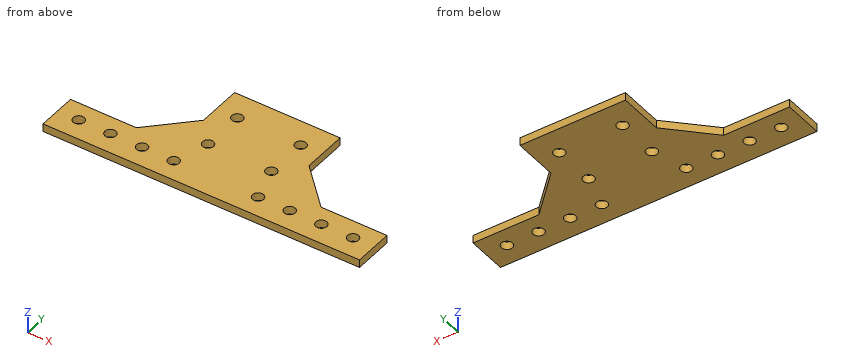
```python
from build123d import *

# Parameters (mm, degrees)
EXTRUDE_1_DEPTH     = 3
SKETCH_2_R          = 2.1
CUT_EXTRUDE_1_DEPTH = 129.910821889


with BuildPart() as part:
    # 草图1 → 凸台-拉伸1 (new body)
    with BuildSketch(Plane.XY):
        Polygon((0, 0), (0, 15), (25, 15), (40, 30), (40, 47), (80, 47), (80, 30), (95, 15), (120, 15), (120, 0), align=None)
    extrude(amount=EXTRUDE_1_DEPTH)

    # 草图2 → 切除-拉伸1 (cut, through all)
    with BuildSketch(Plane.XY.offset(3)):
        with Locations((48, 37)):
            Circle(SKETCH_2_R)
        with Locations((72, 37)):
            Circle(SKETCH_2_R)
        with Locations((48, 21)):
            Circle(SKETCH_2_R)
        with Locations((72, 21)):
            Circle(SKETCH_2_R)
        with Locations((112, 8)):
            Circle(SKETCH_2_R)
        with Locations((76, 8)):
            Circle(SKETCH_2_R)
        with Locations((88, 8)):
            Circle(SKETCH_2_R)
        with Locations((8, 8)):
            Circle(SKETCH_2_R)
        with Locations((20, 8)):
            Circle(SKETCH_2_R)
        with Locations((100, 8)):
            Circle(SKETCH_2_R)
        with Locations((32, 8)):
            Circle(SKETCH_2_R)
        with Locations((44, 8)):
            Circle(SKETCH_2_R)
        with Locations((432, 8)):
            Circle(SKETCH_2_R)
        with Locations((444, 8)):
            Circle(SKETCH_2_R)
        with Locations((524, 8)):
            Circle(SKETCH_2_R)
        with Locations((536, 8)):
            Circle(SKETCH_2_R)
        with Locations((456, 8)):
            Circle(SKETCH_2_R)
        with Locations((468, 8)):
            Circle(SKETCH_2_R)
        with Locations((500, 8)):
            Circle(SKETCH_2_R)
        with Locations((512, 8)):
            Circle(SKETCH_2_R)
    extrude(amount=-CUT_EXTRUDE_1_DEPTH, mode=Mode.SUBTRACT)


solid = part.part
```
Design review of the part built by this model. Coordinates are the model's own, in mm. Give positions to 0.01 mm unless a question says otherwise; leave off trailing zeros. Write each loop counter-clockwise with the first axis right and the second up, starting at its lowest first coordinate (ties: lowest second). Pieces come first, ordered by that corner, then holes.
(1) Wall thickness on line 1 along Y through (x, z) = (48, 1.9); line 2 along Y through (x, z) = (95, 0.2); line 3 along X through (y, z) = (42, 2.4): over which ranges is each line inside the solid? List them lowest first.
Checked values:
line 1: y = 0 to 18.9, 23.1 to 34.9, 39.1 to 47
line 2: y = 0 to 15
line 3: x = 40 to 80
(2) Add section A-A (x = 100). Give the boundary of the cut face in (y, z), and give its area (3 significant figures).
Checked values:
outline: (0, 0) - (5.9, 0) - (5.9, 3) - (0, 3) - close; (10.1, 0) - (15, 0) - (15, 3) - (10.1, 3) - close
area: 32.4 mm2
(3) Add section C-C (z = 1.35). Give the number of separate pieces and of enclosed holes in the cut face, and give its area (3 significant figures).
Checked values:
separate pieces: 1
enclosed holes: 12
area: 3,140 mm2
(4) Add section B-B (y = 21). Give the boundary of the cut face in (x, z).
Checked values:
outline: (31, 0) - (45.9, 0) - (45.9, 3) - (31, 3) - close; (50.1, 0) - (69.9, 0) - (69.9, 3) - (50.1, 3) - close; (74.1, 0) - (89, 0) - (89, 3) - (74.1, 3) - close
(5) Clearance check with flat-ended pins moving along their axes: pin 1 Ø0.9 at (y, z) = (40.5, 2) entering from +X; pin 2 Ø0.9 at (x, z) = (11, 1.5) entering from +Y; pin 3 Ø0.9 at (y, z) = (36.5, 1) entering from -X. State where each tip first meets the part, or that it passes through.
Checked values:
pin 1: stops at x = 80
pin 2: stops at y = 15
pin 3: stops at x = 40
